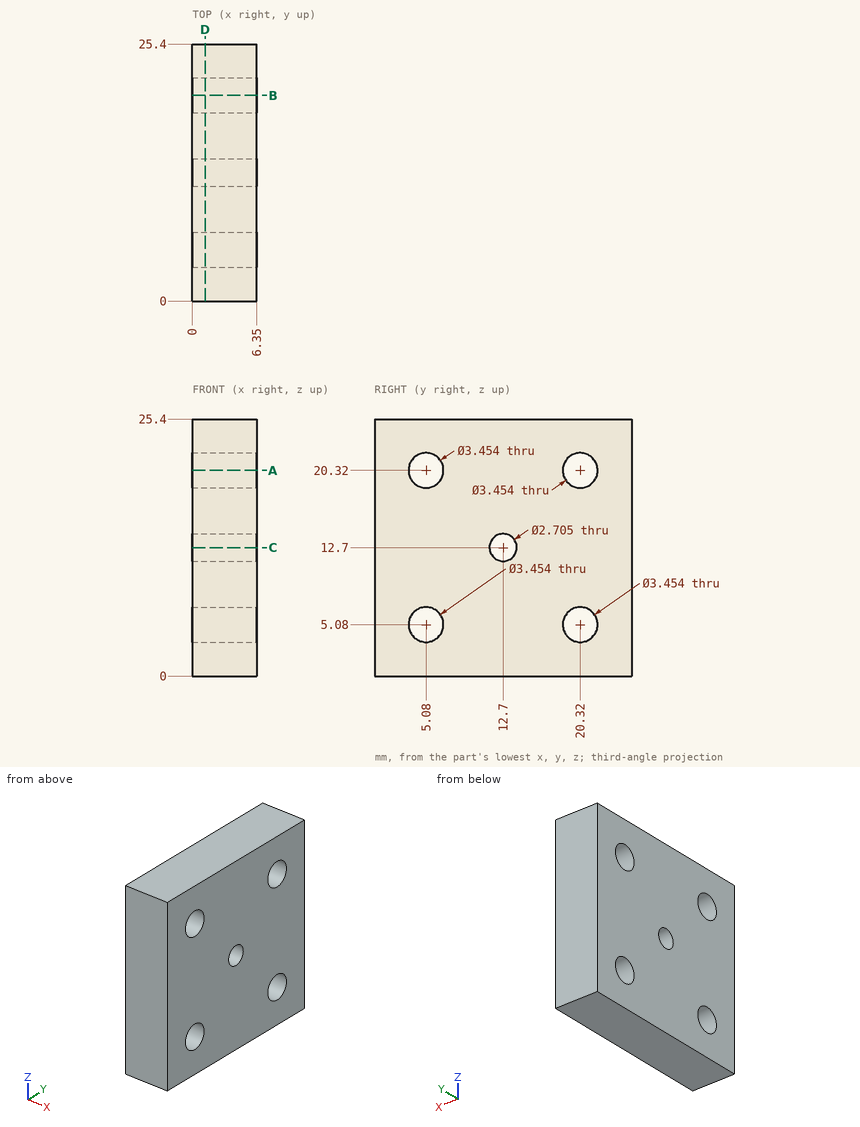
The figure shows three views and two pictorial views of one solid part (mm, origin at its lowest corner). Answer the questions. Coordinates: 2 decimals unless noted, no trailing zeros. Loops run counter-clockwise (first coordinate to the right, second up) from the corner with the lowest first, then second, coordinate; pieces in that order, holes last.
1) Find section D-D on x = 1.25. Write down the section's boundary in (y, z) (1 decimal), then the cut area to 3 significant figures.
2) Find section A-A on z = 20.32. Write down the section's boundary in (x, y).
3) Find section C-C on z = 12.7. Write down the section's boundary in (x, y), then the cut area to 3 significant figures.
4) Find the intervals of material crossed by L1, parallel to Z at x = 3, y = 5 (1 decimal); L2, parallel to Y at x = 2.5, z = 5.08; L3, parallel to Y at x = 3.5, z = 12.7, in increasing order.
5) A flat-ended cylindrical pin translates along its axis: pin 1 Ø3 at (y, z) = (5.08, 5.08) entering from +X. Find the tip coordinate at first contact, or state that the pin passes through.
Values:
1. outline: (0, 0) - (25.4, 0) - (25.4, 25.4) - (0, 25.4) - close; hole circle Ø3.5 at (5.1, 5.1); hole circle Ø3.5 at (5.1, 20.3); hole circle Ø2.7 at (12.7, 12.7); hole circle Ø3.5 at (20.3, 5.1); hole circle Ø3.5 at (20.3, 20.3)
1. area: 602 mm2
2. outline: (0, 0) - (6.35, 0) - (6.35, 3.35) - (0, 3.35) - close; (0, 6.81) - (6.35, 6.81) - (6.35, 18.59) - (0, 18.59) - close; (0, 22.05) - (6.35, 22.05) - (6.35, 25.4) - (0, 25.4) - close
3. outline: (0, 0) - (6.35, 0) - (6.35, 11.35) - (0, 11.35) - close; (0, 14.05) - (6.35, 14.05) - (6.35, 25.4) - (0, 25.4) - close
3. area: 144 mm2
4. L1: z = 0 to 3.4, 6.8 to 18.6, 22 to 25.4
4. L2: y = 0 to 3.35, 6.81 to 18.59, 22.05 to 25.4
4. L3: y = 0 to 11.35, 14.05 to 25.4
5. pin 1: passes through
